For this review, take the finished solid that the model builds, in its own axes (mm). A direction names the side the tool comes from. Give positions to 0.01 mm unless a question says otherwise; leave off trailing zeros. Write each loop counter-clockwise with the first axis right and the second up, starting at its lowest first coordinate (ties: lowest second). Pieces come first, ordered by that corner, then holes. Notation, with made-up numbers: M 22.5,12 L 43.5,12 A19 cw 43.5,43 Z; hole C 0.5,-34 d11. An arc over 180 degrees is marked long. Use one line per item in the form item = value. Start each with the question number.
Q1. Clearance check with flat-ended pins moving along their axes: pin 1 Ø5.5 at (x, y) = (10, 5) entering from +Z; pin 2 Ø4 at (x, y) = (-19, 21.5) entering from -Z; pin 3 Ø5 at (x, z) = (-32.5, -0.5) entering from +Y. State where each tip first meets the part, or that it passes through.
Q2. Mouldability with a two-part tool opening along Y and no side actions: class faces 1 (the flat face through (-0.1, 2.4, -11.78)), 2 (the cylindrical face through (16.665, 5.341, 10.493)) as released by +Y, released by -Y, zero draft, split by the parting line, or undercut.
Q3. Consider section B-B on x = 38.5. Write out the cut boundary in (y, z), and give its area (3 significant figures).
Q4. Tool access review of faces 3 (the flat face through (4.656, 10.662, -10.507)), 4 (the flat face through (-4.7, 10.72, 10.49)): name each direction out of +Z, -Z, +X, -X, +Y, -Y from which nothing blocks a thin tool from reaching the whole face with its end or side.
Q5. For probe 1 along Y at (x, z) = (0, 0); probe 2 along Z at (x, y) = (3.5, -24); probe 3 along X at (y, z) = (-1, -7.5), list the stretches that pass through material, from the lowest coordinate up. Write a range as [from, to].
Q6. Consider section A-A on z = 5.5. Write out the cut boundary in (x, y), and give its area (3 significant figures).
```python
from build123d import *
from build123d.topology import SkipClean

# Parameters (mm, degrees)
SKETCH1_R                = 44.45
SKETCH1_R_2              = 2
BOSS_EXTRUDE1_DEPTH      = 11
BOSS_EXTRUDE3_START      = 0.5
SKETCH3_R                = 21.25
SKETCH3_R_2              = 2
BOSS_EXTRUDE3_DEPTH      = 0.5
CUT_EXTRUDE1_DEPTH       = 1.5
FILLET1_R                = 2.5
CIRPATTERN1_COUNT        = 5
FILLET1_OF_CIRPATTERN1_R = 2.5
SKETCH5_R                = 19.45
CUT_EXTRUDE2_DEPTH       = 0.5
BOSS_EXTRUDE4_START      = 0.78
SKETCH6_R                = 5.5
SKETCH6_R_2              = 2
BOSS_EXTRUDE4_DEPTH      = 0.78
MIRROR1_START            = 10
MIRROR1_DEPTH            = 1
MIRROR1_START_2          = 11
MIRROR1_2_OUTLINE_R      = 21.25
MIRROR1_2_OUTLINE_R_2    = 19.45
MIRROR1_2_OUTLINE_R_3    = 5.5
MIRROR1_2_OUTLINE_R_4    = 2
MIRROR1_2_DEPTH          = 0.5
MIRROR1_START_3          = 11.5
MIRROR1_3_OUTLINE_R      = 5.5
MIRROR1_3_OUTLINE_R_2    = 2
MIRROR1_3_DEPTH          = 0.28


# Read off the part's stored shape, not the designer's step: Mirror1
with BuildPart() as part:
    # Sketch1 → Boss-Extrude1 (new, symmetric)
    with BuildSketch(Plane.XY):
        Circle(SKETCH1_R)
        Circle(SKETCH1_R_2, mode=Mode.SUBTRACT)
    extrude(amount=BOSS_EXTRUDE1_DEPTH, both=True)

    # Sketch3 → Boss-Extrude3 (add)
    with SkipClean():  # the faces are left unmerged after this step: merging them gives an invalid solid
        with BuildSketch(Plane(origin=(0, 0, -11), x_dir=(-1, 0, 0), z_dir=(0, 0, -1)).offset(BOSS_EXTRUDE3_START)):
            with Locations(Location((0, 0, 0), (0, 0, 180))):
                Circle(SKETCH3_R)
            Circle(SKETCH3_R_2, mode=Mode.SUBTRACT)
        extrude(amount=-BOSS_EXTRUDE3_DEPTH)

    # Sketch4 → Cut-Extrude1 (cut)
    with SkipClean():  # the faces are left unmerged after this step: merging them gives an invalid solid
        with BuildSketch(Plane(origin=(0, 0, -11.5), x_dir=(-1, 0, 0), z_dir=(0, 0, -1))):
            with BuildLine():
                Line((8.158196723, 15.482048515), (2.133726892, 7.190077159))
                ThreePointArc((2.133726892, 7.190077159), (0, 7.5), (-2.133726892, 7.190077159))
                Line((-2.133726892, 7.190077159), (-8.158196723, 15.482048515))
                ThreePointArc((-8.158196723, 15.482048515), (0, 17.5), (8.158196723, 15.482048515))
            make_face()
        cut_extrude1 = extrude(amount=-CUT_EXTRUDE1_DEPTH, mode=Mode.SUBTRACT)

    # Fillet1
    fillet1_edges = [part.edges().sort_by_distance(p)[0] for p in [
        (8.158196723, 15.482048515, -10.75),
        (-8.158196723, 15.482048515, -10.75),
        (-2.133726892, 7.190077159, -10.75),
        (2.133726892, 7.190077159, -10.75),
    ]]
    fillet(fillet1_edges, radius=FILLET1_R)

    # CirPattern1: Cut-Extrude1 ×5 about axis
    cirpattern1_axis = Axis((0, 0, 0), (0, 0, 1))
    for i in range(1, CIRPATTERN1_COUNT):
        add(cut_extrude1.rotate(cirpattern1_axis, i * 360 / CIRPATTERN1_COUNT), mode=Mode.SUBTRACT)

    # Fillet1 of CirPattern1
    fillet1_of_cirpattern1_edges = [part.edges().sort_by_distance(p)[0] for p in [
        (-12.203281695, 12.543122254, -10.75),
        (-17.245324557, -2.974690056, -10.75),
        (-7.497527606, 0.192561168, -10.75),
        (-6.178811864, 4.251150897, -10.75),
        (-15.700239585, -7.729972637, -10.75),
        (-2.5, -17.320508076, -10.75),
        (-2.5, -7.071067812, -10.75),
        (-5.952442634, -4.562721413, -10.75),
        (2.5, -17.320508076, -10.75),
        (15.700239585, -7.729972637, -10.75),
        (5.952442634, -4.562721413, -10.75),
        (2.5, -7.071067812, -10.75),
        (17.245324557, -2.974690056, -10.75),
        (12.203281695, 12.543122254, -10.75),
        (6.178811864, 4.251150897, -10.75),
        (7.497527606, 0.192561168, -10.75),
    ]]
    fillet(fillet1_of_cirpattern1_edges, radius=FILLET1_OF_CIRPATTERN1_R)

    # Sketch5 → Cut-Extrude2 (cut)
    with BuildSketch(Plane(origin=(0, 0, -11.5), x_dir=(-1, 0, 0), z_dir=(0, 0, -1))):
        Circle(SKETCH5_R)
    extrude(amount=-CUT_EXTRUDE2_DEPTH, mode=Mode.SUBTRACT)

    # Sketch6 → Boss-Extrude4 (add)
    with BuildSketch(Plane(origin=(0, 0, -11), x_dir=(-1, 0, 0), z_dir=(0, 0, -1)).offset(BOSS_EXTRUDE4_START)):
        with Locations(Location((0, 0, 0), (0, 0, 180))):
            Circle(SKETCH6_R)
        Circle(SKETCH6_R_2, mode=Mode.SUBTRACT)
    extrude(amount=-BOSS_EXTRUDE4_DEPTH)

    # Mirror1 outline → Mirror1 (cut)
    with BuildSketch(Plane.XY.offset(MIRROR1_START)):
        with BuildLine():
            Line((-7.46384855, -5.053806964), (-12.677427753, -6.747801535))
            ThreePointArc((-12.677427753, -6.747801535), (-14.292248864, -8.383489285), (-13.889032812, -10.646349964))
            ThreePointArc((-13.889032812, -10.646349964), (-10.286241915, -14.157797402), (-5.833333333, -16.499158228))
            ThreePointArc((-5.833333333, -16.499158228), (-3.556624327, -16.183377076), (-2.5, -14.142135624))
            Line((-2.5, -14.142135624), (-2.5, -8.660254038))
            ThreePointArc((-2.5, -8.660254038), (-2.834936491, -7.410254038), (-3.75, -6.495190528))
            ThreePointArc((-3.75, -6.495190528), (-4.408389392, -6.067627458), (-5.018479548, -5.573586191))
            ThreePointArc((-5.018479548, -5.573586191), (-6.171526837, -4.986079253), (-7.46384855, -5.053806964))
        make_face()
        with BuildLine():
            ThreePointArc((5.018479548, -5.573586191), (4.408389392, -6.067627458), (3.75, -6.495190528))
            ThreePointArc((3.75, -6.495190528), (2.834936491, -7.410254038), (2.5, -8.660254038))
            Line((2.5, -8.660254038), (2.5, -14.142135624))
            ThreePointArc((2.5, -14.142135624), (3.556624327, -16.183377076), (5.833333333, -16.499158228))
            ThreePointArc((5.833333333, -16.499158228), (10.286241915, -14.157797402), (13.889032812, -10.646349964))
            ThreePointArc((13.889032812, -10.646349964), (14.292248864, -8.383489285), (12.677427753, -6.747801535))
            Line((12.677427753, -6.747801535), (7.46384855, -5.053806964))
            ThreePointArc((7.46384855, -5.053806964), (6.171526837, -4.986079253), (5.018479548, -5.573586191))
        make_face()
        with BuildLine():
            ThreePointArc((6.851590932, 3.050524823), (7.132923872, 2.317627458), (7.336107006, 1.559337681))
            ThreePointArc((7.336107006, 1.559337681), (7.923613944, 0.406290392), (9.008933521, -0.298524383))
            Line((9.008933521, -0.298524383), (14.222512725, -1.992518954))
            ThreePointArc((14.222512725, -1.992518954), (16.490363583, -1.618387801), (17.49423108, 0.449309393))
            ThreePointArc((17.49423108, 0.449309393), (16.643489035, 5.407797401), (14.417227682, 9.919352094))
            ThreePointArc((14.417227682, 9.919352094), (12.389719901, 11.002095754), (10.335081241, 9.971764926))
            Line((10.335081241, 9.971764926), (7.11291209, 5.536829561))
            ThreePointArc((7.11291209, 5.536829561), (6.649149838, 4.328687589), (6.851590932, 3.050524823))
        make_face()
        with BuildLine():
            ThreePointArc((-0.783963475, 7.458914215), (0, 7.5), (0.783963475, 7.458914215))
            ThreePointArc((0.783963475, 7.458914215), (2.062126241, 7.66135531), (3.067827119, 8.475755823))
            Line((3.067827119, 8.475755823), (6.28999627, 12.910691187))
            ThreePointArc((6.28999627, 12.910691187), (6.634980854, 15.183158408), (4.978696081, 16.776846704))
            ThreePointArc((4.978696081, 16.776846704), (0, 17.5), (-4.978696081, 16.776846704))
            ThreePointArc((-4.978696081, 16.776846704), (-6.634980854, 15.183158408), (-6.28999627, 12.910691187))
            Line((-6.28999627, 12.910691187), (-3.067827119, 8.475755823))
            ThreePointArc((-3.067827119, 8.475755823), (-2.062126241, 7.66135531), (-0.783963475, 7.458914215))
        make_face()
        with BuildLine():
            ThreePointArc((-7.336107006, 1.559337681), (-7.132923872, 2.317627458), (-6.851590932, 3.050524823))
            ThreePointArc((-6.851590932, 3.050524823), (-6.649149838, 4.328687589), (-7.11291209, 5.536829561))
            Line((-7.11291209, 5.536829561), (-10.335081241, 9.971764926))
            ThreePointArc((-10.335081241, 9.971764926), (-12.389719901, 11.002095754), (-14.417227682, 9.919352094))
            ThreePointArc((-14.417227682, 9.919352094), (-16.643489035, 5.407797401), (-17.49423108, 0.449309393))
            ThreePointArc((-17.49423108, 0.449309393), (-16.490363583, -1.618387801), (-14.222512725, -1.992518954))
            Line((-14.222512725, -1.992518954), (-9.008933521, -0.298524383))
            ThreePointArc((-9.008933521, -0.298524383), (-7.923613944, 0.406290392), (-7.336107006, 1.559337681))
        make_face()
    extrude(amount=MIRROR1_DEPTH, mode=Mode.SUBTRACT)

    # Mirror1 2 outline → Mirror1 2 (add)
    # profile 1 of 2: a face of its own
    with BuildSketch(Plane.XY.offset(MIRROR1_START_2)):
        Circle(MIRROR1_2_OUTLINE_R)
        Circle(MIRROR1_2_OUTLINE_R_2, mode=Mode.SUBTRACT)
    # profile 2 of 2: a face of its own
    with BuildSketch(Plane.XY.offset(MIRROR1_START_2)):
        Circle(MIRROR1_2_OUTLINE_R_3)
        Circle(MIRROR1_2_OUTLINE_R_4, mode=Mode.SUBTRACT)
    extrude(amount=MIRROR1_2_DEPTH)

    # Mirror1 3 outline → Mirror1 3 (add)
    with BuildSketch(Plane.XY.offset(MIRROR1_START_3)):
        Circle(MIRROR1_3_OUTLINE_R)
        Circle(MIRROR1_3_OUTLINE_R_2, mode=Mode.SUBTRACT)
    extrude(amount=MIRROR1_3_DEPTH)


solid = part.part
```
Working result:
q1.pin_1 = 11
q1.pin_2 = -11
q1.pin_3 = 32.8
q2.face_1 = zero draft
q2.face_2 = undercut
q3.outline = M -22.22,-11 L 22.22,-11 L 22.22,11 L -22.22,11 Z
q3.area = 978 mm²
q4.face_3 = -Z
q4.face_4 = +Z
q5.probe_1 = [-44.45, -2], [2, 44.45]
q5.probe_2 = [-11, 11]
q5.probe_3 = [-44.44, -1.73], [1.73, 44.44]
q6.outline = C 0,0 d88.9; hole C 0,0 d4
q6.area = 6,190 mm²
